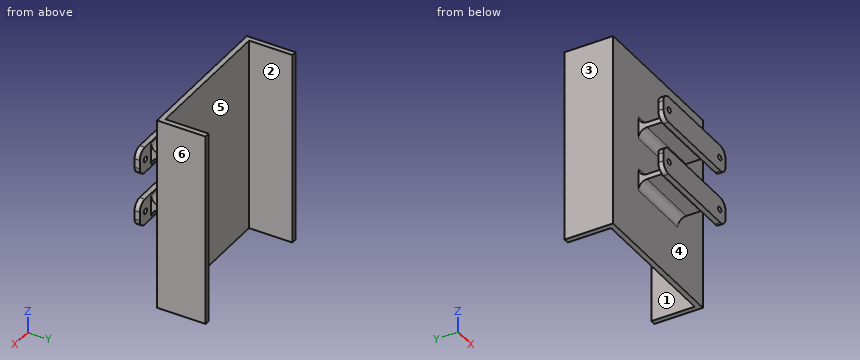
```python
from build123d import *

# Parameters (mm, degrees)
SKETCH1_W             = 87
SKETCH1_H             = 112
BOSS_EXTRUDE1_DEPTH   = 3
SKETCH2_W             = 38
SKETCH2_H             = 3
BOSS_EXTRUDE2_DEPTH   = 18
SKETCH8_W             = 60
SKETCH8_H             = 15
SKETCH8_R             = 1.575
SKETCH8_W_2           = 38
SKETCH8_H_2           = 3
BOSS_EXTRUDE5_DEPTH   = 3
BOSS_EXTRUDE5_2_DEPTH = 3
SKETCH9_W             = 38
SKETCH9_H             = 3
BOSS_EXTRUDE6_DEPTH   = 3
SKETCH10_W            = 38
SKETCH10_H            = 3
BOSS_EXTRUDE7_DEPTH   = 3
FILLET2_R             = 5
FILLET3_R             = 5
FILLET4_R             = 5
SKETCH12_W            = 3
SKETCH12_H            = 112
BOSS_EXTRUDE8_DEPTH   = 25


with BuildPart() as part:
    # Sketch1 → Boss-Extrude1 (new body)
    with BuildSketch(Plane(origin=(0, 0, 0), x_dir=(1, 0, 0), z_dir=(0, 1, 0))):
        Rectangle(SKETCH1_W, SKETCH1_H)
    extrude(amount=BOSS_EXTRUDE1_DEPTH)

    # Sketch2 → Boss-Extrude2 (add)
    with BuildSketch(Plane.XZ):
        with Locations((0, -15.5)):
            Rectangle(SKETCH2_W, SKETCH2_H)
        with Locations((0, 15.5)):
            Rectangle(SKETCH2_W, SKETCH2_H)
    extrude(amount=BOSS_EXTRUDE2_DEPTH)



with BuildPart() as body_2:
    # Sketch8 → Boss-Extrude5 (new body)
    with BuildSketch(Plane.XZ.offset(18)):
        with Locations((0, 15.5)):
            Rectangle(SKETCH8_W, SKETCH8_H)
        with Locations(Location((-24.5, 15.5, 0), (0, 0, 270))):
            Circle(SKETCH8_R, mode=Mode.SUBTRACT)
        with Locations(Location((24.5, 15.5, 0), (0, 0, 90))):
            Circle(SKETCH8_R, mode=Mode.SUBTRACT)
        with Locations((0, 15.5)):
            Rectangle(SKETCH8_W_2, SKETCH8_H_2, mode=Mode.SUBTRACT)
    extrude(amount=BOSS_EXTRUDE5_DEPTH)


with BuildPart() as body_3:
    # Sketch8 → Boss-Extrude5 2 (new body)
    with BuildSketch(Plane.XZ.offset(18)):
        with Locations((0, -15.5)):
            Rectangle(SKETCH8_W, SKETCH8_H)
        with Locations(Location((-24.5, -15.5, 0), (0, 0, 270))):
            Circle(SKETCH8_R, mode=Mode.SUBTRACT)
        with Locations(Location((24.5, -15.5, 0), (0, 0, 90))):
            Circle(SKETCH8_R, mode=Mode.SUBTRACT)
        with Locations((0, -15.5)):
            Rectangle(SKETCH8_W_2, SKETCH8_H_2, mode=Mode.SUBTRACT)
    extrude(amount=BOSS_EXTRUDE5_2_DEPTH)


with BuildPart() as part_1:
    add(part.part)

    add(body_2.part)  # Boss-Extrude6 merges body 2
    # Sketch9 → Boss-Extrude6 (add)
    with BuildSketch(Plane.XY.offset(14)):
        with Locations((0, -19.5)):
            Rectangle(SKETCH9_W, SKETCH9_H)
    extrude(amount=BOSS_EXTRUDE6_DEPTH)


    add(body_3.part)  # Boss-Extrude7 merges body 3
    # Sketch10 → Boss-Extrude7 (add)
    with BuildSketch(Plane(origin=(0, 0, -14), x_dir=(-1, 0, 0), z_dir=(0, 0, -1))):
        with Locations((0, -19.5)):
            Rectangle(SKETCH10_W, SKETCH10_H)
    extrude(amount=BOSS_EXTRUDE7_DEPTH)

    # Fillet2
    fillet2_edges = [part_1.edges().sort_by_distance(p)[0] for p in [
        (-30, -19.5, -8),
        (30, -19.5, -8),
        (30, -19.5, -23),
        (-30, -19.5, -23),
    ]]
    fillet(fillet2_edges, radius=FILLET2_R)

    # Fillet3
    fillet3_edges = [part_1.edges().sort_by_distance(p)[0] for p in [
        (-30, -19.5, 23),
        (-30, -19.5, 8),
        (30, -19.5, 8),
        (30, -19.5, 23),
    ]]
    fillet(fillet3_edges, radius=FILLET3_R)

    # Fillet4
    fillet4_edges = [part_1.edges().sort_by_distance(p)[0] for p in [
        (0, 0, 14),
        (0, 0, 17),
        (0, 0, -14),
        (0, 0, -17),
        (0, -18, -14),
        (0, -18, -17),
        (0, -18, 17),
        (0, -18, 14),
    ]]
    fillet(fillet4_edges, radius=FILLET4_R)

    # Sketch12 → Boss-Extrude8 (add)
    with BuildSketch(Plane(origin=(0, 3, 0), x_dir=(1, 0, 0), z_dir=(0, 1, 0))):
        with Locations((42, 0)):
            Rectangle(SKETCH12_W, SKETCH12_H)
        with Locations((-42, 0)):
            Rectangle(SKETCH12_W, SKETCH12_H)
    extrude(amount=BOSS_EXTRUDE8_DEPTH)


solid = part_1.part
```
Could you check a few things on this model? Use its own coordinates, in mm. Face numbers are marked on the shaded views. A direction names the side the tool comes from. Round coordinates to 2 decimals unless told otherwise and drop trailing zeros. Write each loop counter-clockwise with the first axis right and the second up, starting at its lowest first coordinate (ties: lowest second). Pieces come first, ordered by that corner, then holes.
(1) Suppose I cut it at A-A on y = 16.5. Write out the boundary of the cut face in (x, z), and give its area (3 significant figures).
Findings below:
outline: (-43.5, -56) - (-40.5, -56) - (-40.5, 56) - (-43.5, 56) - close; (40.5, -56) - (43.5, -56) - (43.5, 56) - (40.5, 56) - close
area: 672 mm2
(2) Which directions (+Z, -Z, +X, -X, +Y, -Y) give clear straight access to the entire face, cutting with the end or side of a thin tool? Please do the marked faces 5 and 6.
Findings below:
face 5: +Z, -Z, +Y
face 6: +Z, -Z, +X, +Y, -Y
(3) If I drill on probe 1 along Z at (x, y) = (24.5, -19.9) (3 decimals); probe 2 along X at (y, z) = (-20.4, 15.5) (3 decimals); probe 3 along Z at (x, y) = (24, -19), over which ranges is the centre line in solid material (lowest first)?
Findings below:
probe 1: z = -23 to -17.075, -13.925 to -8, 8 to 13.925, 17.075 to 23
probe 2: x = -30 to -26.075, -22.925 to 22.925, 26.075 to 30
probe 3: z = -23 to -16.99, -14.01 to -8, 8 to 14.01, 16.99 to 23
(4) Suppose I cut it at C-C on x = 15. Write out the boundary of the cut face in (y, z), and give its area (3 significant figures).
Findings below:
outline: (-21, -23) - (-18, -23) - (-18, -22) arc R5 cw to (-13, -17) - (-5, -17) arc R5 cw to (0, -22) - (0, -56) - (3, -56) - (3, 56) - (0, 56) - (0, 22) arc R5 cw to (-5, 17) - (-13, 17) arc R5 cw to (-18, 22) - (-18, 23) - (-21, 23) - (-21, 8) - (-18, 8) - (-18, 9) arc R5 cw to (-13, 14) - (-5, 14) arc R5 cw to (0, 9) - (0, -9) arc R5 cw to (-5, -14) - (-13, -14) arc R5 cw to (-18, -9) - (-18, -8) - (-21, -8) - close
area: 577 mm2
(5) Thinking about a two-plate mould opening in X: for the marked faces 1, 2, 3 and 4, which applies, +X half, -X half, draft (parallel to the pull), parting line (faces both ways), or undercut?
Findings below:
face 1: undercut
face 2: undercut
face 3: -X half
face 4: draft
(6) For pin 1 (3 mm diameter, centred on x = 24.5, z = 15.5, fed in from +Y); pin 2 (3.5 mm diameter, centred on y = -20, z = 16.5, fed in from +X); pin 3 (9 mm diameter, centred on x = -4.5, y = -10.5, fed in from +Z), each with a flat end and sliding along its axis, tell me the tip position at first contact or that it passes through.
Findings below:
pin 1: stops at y = 3
pin 2: stops at x = 30
pin 3: stops at z = 17.42
(7) Suppose I cut it at B-B on z = 15.5. Write out the boundary of the cut face in (x, y) (3 decimals).
Findings below:
outline: (-43.5, 0) - (-19, 0) - (-19, -18) - (-22.925, -18) - (-22.925, -21) - (22.925, -21) - (22.925, -18) - (19, -18) - (19, 0) - (43.5, 0) - (43.5, 28) - (40.5, 28) - (40.5, 3) - (-40.5, 3) - (-40.5, 28) - (-43.5, 28) - close; (-30, -21) - (-26.075, -21) - (-26.075, -18) - (-30, -18) - close; (26.075, -21) - (30, -21) - (30, -18) - (26.075, -18) - close
(8) Suppose I cut it at D-D on z = -0.5. Write out the boundary of the cut face in (x, y).
Findings below:
outline: (-43.5, 0) - (43.5, 0) - (43.5, 28) - (40.5, 28) - (40.5, 3) - (-40.5, 3) - (-40.5, 28) - (-43.5, 28) - close
